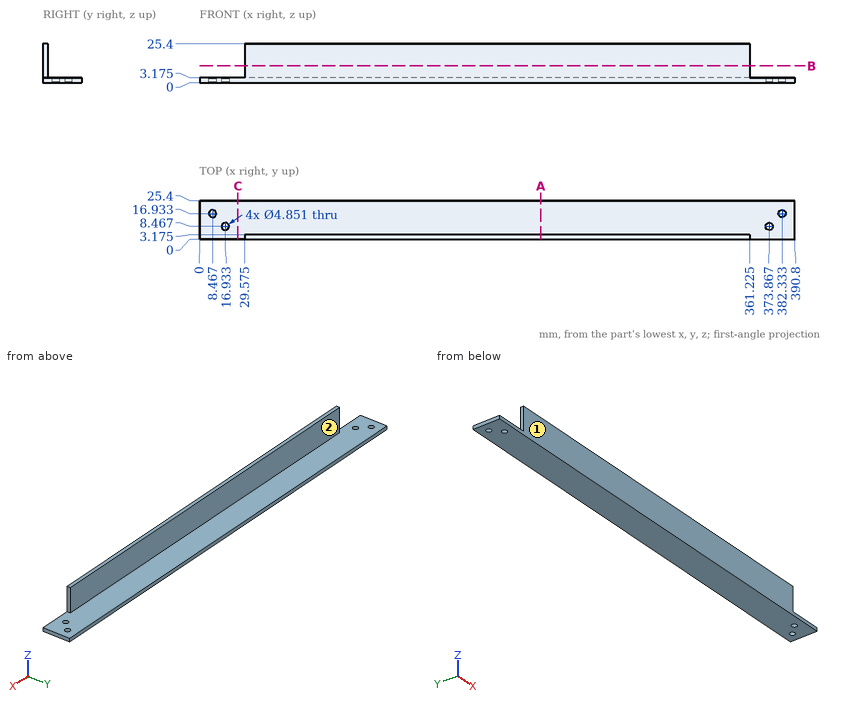
Input: dimensioned drawing with shaded views. Units: mm. Origin: part minimum x, y, z. A direction names the side the tool comes from. Coordinates: 2 decimals unless noted, no trailing zeros. Order: outer loops, then holes, each group sorted by start corner. A loop starts at its lowest first (then second) coordinate and runs counter-clockwise, first axis right, second up.
(1) Access query for the marked faces 1 and 2. Directions: +Z, -Z, +X, -X, +Y, -Y. A direction counts if a zero-diameter tool reaches every point of the face in a straight line with its end or side. Return the directions, or none.
(2) First-contact query: pin 1 (6 mm diameter, centred on x = 262.5, z = 12, fed in from +Y) (3 decimals); pin 2 (6 mm diameter, centred on x = 152, y = 8.5, fed in from +Z) (3 decimals); pin 3 (3 mm diameter, centred on x = 8.47, y = 16.93, fed in from -Z); pin 4 (1.6 mm diameter, centred on y = 1, z = 14.5, fed in from +X) (3 decimals). Flat tips, straight axial feed; report the tip coordinate or a pass-through.
(3) Section query A-A (x = 224). Return the cut outline in (y, z) (1 decimal), plus the area to 3 significant figures.
(4) Section query B-B (z = 11). Return the cut outline in (x, y) (1 decimal), plus the area to 3 significant figures.
(5) Section query C-C (x = 25). Return the cut outline in (y, z) (1 decimal).
(6) Material intervals for probe 1 along Y at (x, z) = (112, 6.5) (1 decimal); probe 2 along X at (y, z) = (2.5, 15) (1 decimal), sorted ascending.
Solution:
1. face 1: +Z, -Z, +X, -X, -Y
1. face 2: +Z, +X, -X, +Y
2. pin 1: stops at y = 3.175
2. pin 2: stops at z = 3.175
2. pin 3: passes through
2. pin 4: stops at x = 361.225
3. outline: (0, 0) - (25.4, 0) - (25.4, 3.2) - (3.2, 3.2) - (3.2, 25.4) - (0, 25.4) - close
3. area: 151 mm2
4. outline: (29.6, 0) - (361.2, 0) - (361.2, 3.2) - (29.6, 3.2) - close
4. area: 1,050 mm2
5. outline: (0, 0) - (25.4, 0) - (25.4, 3.2) - (0, 3.2) - close
6. probe 1: y = 0 to 3.2
6. probe 2: x = 29.6 to 361.2
